```python
from build123d import *

# Parameters (mm, degrees)
SKETCH1_R           = 1
BOSS_EXTRUDE1_DEPTH = 1.5


with BuildPart() as part:
    # Sketch1 → Boss-Extrude1 (new body)
    with BuildSketch(Plane(origin=(0, 0, 0), x_dir=(1, 0, 0), z_dir=(0, 1, 0))):
        with BuildLine():
            Line((0, 0), (20, 0))
            Line((20, 0), (20, 10))
            Line((20, 10), (27, 10))
            Line((27, 10), (27, 0))
            Line((27, 0), (27, -2.5))
            Line((27, -2.5), (37.817581496, -2.5))
            ThreePointArc((37.817581496, -2.5), (32.861344207, -7.249817199), (27, -10.823288281))
            ThreePointArc((27, -10.823288281), (13.5, -13.83633472), (0, -10.823288281))
            ThreePointArc((0, -10.823288281), (-5.861344207, -7.249817199), (-10.817581496, -2.5))
            Line((-10.817581496, -2.5), (0, -2.5))
            Line((0, -2.5), (0, 0))
        make_face()
        with Locations(Location((30, -4.881961213, 0), (0, 0, 270))):
            Circle(SKETCH1_R, mode=Mode.SUBTRACT)
        with Locations(Location((-3, -4.881961213, 0), (0, 0, 90))):
            Circle(SKETCH1_R, mode=Mode.SUBTRACT)
    extrude(amount=BOSS_EXTRUDE1_DEPTH)


solid = part.part
```
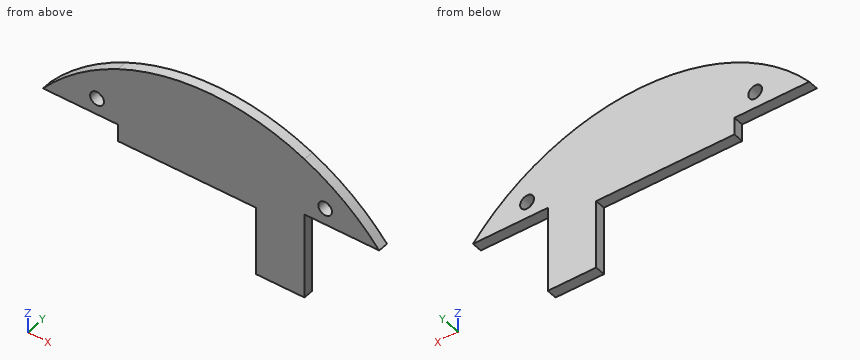
Work out the finished part from the listing and answer in its coordinate system (mm). Give positions to 0.01 mm unless a question says otherwise; leave off trailing zeros. Write each loop counter-clockwise with the first axis right and the second up, starting at its lowest first coordinate (ties: lowest second). Pieces come first, ordered by that corner, then holes.
(1) The part is cut by section B-B on x = -3. Write down the section's boundary in (y, z).
Final values:
outline: (0, 2.5) - (1.5, 2.5) - (1.5, 3.88) - (0, 3.88) - close; (0, 5.88) - (1.5, 5.88) - (1.5, 9.21) - (0, 9.21) - close
(2) The part is cut by section C-C on z = -6.5. Write down the section's boundary in (x, y), plus the area to 3 significant figures.
Final values:
outline: (20, 0) - (27, 0) - (27, 1.5) - (20, 1.5) - close
area: 10.5 mm2
(3) Straight lines are drawn through the part: line 1 (X direction, y = 1.15, z = 4); line 2 (X direction, y = 0.9, z = 4.25) (3 decimals); line 3 (X direction, y = 1.25, z = -1.75). For each, find the intervals that lie inside material, in ascending order.
Final values:
line 1: x = -9.48 to -3.47, -2.53 to 29.53, 30.47 to 36.48
line 2: x = -9.234 to -3.775, -2.225 to 29.225, 30.775 to 36.234
line 3: x = 20 to 27
(4) A flat-ended cylindrical pin translates along its axis: pin 1 Ø1.6 at (x, z) = (30, 4.88) entering from -Y. Find the tip coordinate at first contact, or state that the pin passes through.
Final values:
pin 1: passes through
(5) The part is cut by section A-A on y = 0.75. Write down the section's boundary in (x, z), plus the area to 3 significant figures.
Final values:
outline: (-10.82, 2.5) - (0, 2.5) - (0, 0) - (20, 0) - (20, -10) - (27, -10) - (27, 2.5) - (37.82, 2.5) arc R31.75 ccw to start; hole circle Ø2 at (-3, 4.88); hole circle Ø2 at (30, 4.88)
area: 514 mm2
(6) The part is cut by section D-D on x = 29.5. Write down the section's boundary in (y, z), plus the area to 3 significant figures.
Final values:
outline: (0, 2.5) - (1.5, 2.5) - (1.5, 4.02) - (0, 4.02) - close; (0, 5.75) - (1.5, 5.75) - (1.5, 9.51) - (0, 9.51) - close
area: 7.92 mm2
